```python
from build123d import *

# Parameters (mm, degrees)
SKETCH2_R           = 1
BOSS_EXTRUDE1_DEPTH = 3


with BuildPart() as part:
    # Sketch2 → Boss-Extrude1 (new body)
    with BuildSketch(Plane.XY):
        with BuildLine():
            Line((-5.603408365, 96.42556159), (-5.603408365, 30.425568858))
            ThreePointArc((-5.603408365, 30.425568858), (-4.43183549, 27.597141733), (-1.603408365, 26.425568858))
            Line((-1.603408365, 26.425568858), (41.26721418, 26.425568858))
            ThreePointArc((41.26721418, 26.425568858), (52.597121833, 23.710837368), (61.46641692, 16.156224264))
            Line((61.46641692, 16.156224264), (63.465114175, 13.41553894))
            ThreePointArc((63.465114175, 13.41553894), (64.657533725, 12.331421876), (66.181004174, 11.805863146))
            Line((66.181004174, 11.805863146), (84.187939735, 9.463477264))
            ThreePointArc((84.187939735, 9.463477264), (103.379739296, 5.009808001), (121.325879515, -3.120160731))
            Line((121.325879515, -3.120160731), (122.126093986, -3.582626958))
            ThreePointArc((122.126093986, -3.582626958), (125.162033535, -3.98331921), (127.591695632, -2.119391819))
            Line((127.591695632, -2.119391819), (143.453487011, 25.354036748))
            ThreePointArc((143.453487011, 25.354036748), (143.853088701, 26.318760568), (143.989385396, 27.354036748))
            Line((143.989385396, 27.354036748), (143.989385396, 98.790469349))
            add(Edge.make_bspline(
                [(-5.603408365, 96.42556159), (-5.603408365, 103.460733083), (68.627157279, 109.640132521), (143.989385396, 103.458567417), (143.989385396, 98.790469349)],
                knots=[0, 0, 0, 0, 0.499912399, 1, 1, 1, 1], degree=3))
        make_face()
        with Locations((21.387798276, 72.300241098)):
            Circle(SKETCH2_R, mode=Mode.SUBTRACT)
        with Locations((21.387798276, 53.550235091)):
            Circle(SKETCH2_R, mode=Mode.SUBTRACT)
        with Locations((64.637863533, 36.300090173)):
            Circle(SKETCH2_R, mode=Mode.SUBTRACT)
        with Locations((111.137845658, 28.550051811)):
            Circle(SKETCH2_R, mode=Mode.SUBTRACT)
        with Locations((97.387827206, 76.050038887)):
            Circle(SKETCH2_R, mode=Mode.SUBTRACT)
        with Locations((140.524945013, 32.281066453)):
            Circle(SKETCH2_R, mode=Mode.SUBTRACT)
        with Locations((123.859596668, 0.88165491)):
            Circle(SKETCH2_R, mode=Mode.SUBTRACT)
        with Locations((66.696986614, 15.772443805)):
            Circle(SKETCH2_R, mode=Mode.SUBTRACT)
        with Locations((-0.871175318, 31.157801905)):
            Circle(SKETCH2_R, mode=Mode.SUBTRACT)
        with Locations((-1.603408365, 95.42556159)):
            Circle(SKETCH2_R, mode=Mode.SUBTRACT)
        with Locations((68.896968427, 102.54989148)):
            Circle(SKETCH2_R, mode=Mode.SUBTRACT)
        with Locations((117.399952063, 99.390469349)):
            Circle(SKETCH2_R, mode=Mode.SUBTRACT)
        with Locations((139.989385396, 97.290469349)):
            Circle(SKETCH2_R, mode=Mode.SUBTRACT)
        with Locations((140.524945013, 55.281066453)):
            Circle(SKETCH2_R, mode=Mode.SUBTRACT)
    extrude(amount=BOSS_EXTRUDE1_DEPTH)


solid = part.part
```
Model file for the job. Use its own axes, mm. A direction names the side the tool comes from. Coordinates: 2 decimals unless noted, no trailing zeros. Order: outer loops, then holes, each group sorted by start corner. A loop starts at its lowest first (then second) coordinate and runs counter-clockwise, first axis right, second up. Notation, with made-up numbers: (69, -12) - (102, -12) arc R25 ccw to (102, 23) - close; hole circle Ø8 at (33, 41). An arc over 180 degrees is marked (long way). Return JSON: item names as keys, results as strings. Group by question number.
1) Flat gauge pins, fed straight in: P1, Ø3, axis at x = 64.64, y = 36.3, coming from the -Z side; P2, Ø1.2, axis at x = 139.99, y = 97.29, coming from the -Z side; P3, Ø1, axis at x = 39, z = 1, coming from the -Y side. Where does each tip first touch, or does it go through?
2) Tool access for faces 1 (the flat face through (68, 66, 0)), 2 (the flat face through (20, 26.426, 1)): list every direction of +Z, -Z, +X, -X, +Y, -Y with a clear straight run to the whole face (end or side of a thin tool).
3) Saw through at A-A, the plane z = 2.45. Count the separate pieces of the cut face and the enclosed holes in it, plus the area to 3 significant figures.
4) Saw through at B-B, the plane y = 19. Write the cut outline in (x, z), plus the area to 3 significant figures.
5) Probe line 1 (Y direction, x = 124.5, z = 1.5); line 2 (X direction, y = 76.5, z = 1.4); line 3 (X direction, y = 72, z = 1.5). List the from-to ranges inside material, lowest first. Write a range as from..to.
Values found:
{
 "1": {"P1": "stops at z = 0", "P2": "passes through", "P3": "stops at y = 26.43"},
 "2": {"face 1": "-Z, +X, -X, +Y, -Y", "face 2": "+Z, -Z, -X, -Y"},
 "3": {"separate pieces": "1", "enclosed holes": "14", "area": "13,300 mm²"},
 "4": {"outline": "(59.05, 0) - (139.78, 0) - (139.78, 3) - (59.05, 3) - close", "area": "242 mm²"},
 "5": {"line 1": "y = -4.1..0.11, 1.65..104", "line 2": "x = -5.6..96.49, 98.28..143.99", "line 3": "x = -5.6..20.43, 22.34..143.99"}
}
